Autodesk Inventor part; units mm, degrees
ref_plane "Start plane" through (0, 0, 0) normal (0, 0, 1) x (1, 0, 0)
ref_plane "End plane" through (0, 0, 500) normal (0, 0, 1) x (1, 0, 0)
ref_plane "YZ Plane" through (0, 0, 0) normal (1, 0, 0) x (0, 1, 0)
ref_plane "Start plane" through (0, 0, 0) normal (0, 0, 1) x (1, 0, 0)
ref_plane "End plane" through (0, 0, 500) normal (0, 0, 1) x (1, 0, 0)
sketch "Sketch" plane through (0, 0, 0) normal (0, 0, 1) x (1, 0, 0)
  line L0 (-3, 0.5) -> (-3, 12)
  line L1 (-6, 14) -> (-5, 14)
  line L2 (-6, -6) -> (-6, 14)
  line L3 (-6, -6) -> (14, -6)
  line L4 (14, -5) -> (14, -6)
  line L5 (0.5, -3) -> (12, -3)
  arc A0 (-3, 0.5) -> (0.5, -3) centre (0.5, 0.5) ccw
  arc A1 (-3, 12) -> (-5, 14) centre (-5, 12) ccw
  arc A2 (14, -5) -> (12, -3) centre (12, -5) ccw
  line L6 (0, 18.4971) -> (0, -10.0828) construction
  line L7 (-10.0828, 0) -> (18.4971, 0) construction
  point P0 (-3, -3)
  point P1 (-3, 14)
  point P2 (14, -3)
  dimension "d4" = 20
  dimension "d6" = 20
  dimension "d8" = 3
  dimension "d10" = 3
  dimension "d17" = 3.5
  dimension "d18" = 2
  dimension "d19" = 6
  dimension "d20" = 6
extrude "Body" add sketch "Sketch" along normal up to surface (500 mm away) from surface at 0
sketch "Sketch3" plane through (0, 0, 0) normal (0, 0, 1) x (1, 0, 0)
  line L0 (0, 0) -> (10, 0)
ref_plane "Work Plane10" through (0, 0, 0) normal (0, -1, 0) x (1, 0, 0)
sketch "Sketch4" plane through (0, 0, 0) normal (0, -1, 0) x (1, 0, 0)
  line L0 (-2, 0) -> (12, 0)
  line L1 (-2, 500) -> (12, 500)
  dimension "d24" = 500
equation "\"d4\" = b"
equation "\"d6\" = b"
equation "\"d17\" = R"
equation "\"d18\" = R1"
equation "\"d19\" = ex"
equation "\"d20\" = d19"
equation "\"d11\" = G_L"
equation "\"b\" = 20"
equation "\"ParT\" = 3"
equation "\"R\" = 3.5"
equation "\"R1\" = 2"
equation "\"G_L\" = d24"
equation "\"ex\" = 6"
equation "\"G_OFFSET_START\" = 0"
equation "\"G_OFFSET_END\" = 0"
properties part number "ISO 657-1 - L20x20x3-500" material "Stainless Steel"
Could you check a few things on this model? Use its own coordinates, in mm. A direction names the side the tool comes from. Give positions to 0.01 mm unless a question says otherwise; leave off trailing zeros. Write each loop counter-clockwise with the first axis right and the second up, starting at its lowest first coordinate (ties: lowest second). Pieces come first, ordered by that corner, then holes. Notation, with made-up numbers: (77.5, 48) -> (103.5, 48) arc R17 ccw to (103.5, 65) -> close; hole circle Ø9 at (9.25, 35). An arc over 180 degrees is marked (long way). Answer as a JSON object with one key per item and string values.
Q1. Which directions (+Z, -Z, +X, -X, +Y, -Y) give clear straight access to the entire face, cutting with the end or side of a thin tool? Please do faces 1 (the flat face through (-6, 4, 246)), 2 (the flat face through (6, -3, 246)).
Taken from the geometry:
{"face 1": "+Z, -Z, -X, +Y, -Y", "face 2": "+Z, -Z, +X, +Y"}
Q2. Please list where these lines run through material, in increasing order: L1, parallel to X at y = 0.5, z = 314; L2, parallel to X at y = 12.5, z = 202.5.
Taken from the geometry:
{"L1": "x = -6 to -3", "L2": "x = -6 to -3.06"}
Q3. Suppose I cut it at A-A on z = 36.5. Write out the boundary of the cut face in (x, y).
Taken from the geometry:
{"outline": "(-6, -6) -> (14, -6) -> (14, -5) arc R2 ccw to (12, -3) -> (0.5, -3) arc R3.5 cw to (-3, 0.5) -> (-3, 12) arc R2 ccw to (-5, 14) -> (-6, 14) -> close"}
Q4. Suppose I cut it at B-B on x = 6.5. Write out the boundary of the cut face in (y, z), then the cut area to 3 significant figures.
Taken from the geometry:
{"outline": "(-6, 0) -> (-3, 0) -> (-3, 500) -> (-6, 500) -> close", "area": "1,500 mm²"}
Q5. Will these pins go through, and if not, where does the flat tip stop? pin 1 Ø9 at (x, z) = (4, 369.5) entering from +Y; pin 2 Ø1 at (y, z) = (10.5, 159) entering from +X.
Taken from the geometry:
{"pin 1": "stops at y = -2.85", "pin 2": "stops at x = -3"}
